Check sheet for the modelled part. Datum: model origin and axes. Units: mm. A direction names the side the tool comes from. Give positions to 0.01 mm unless a question says otherwise; leave off trailing zeros. Order: outer loops, then holes, each group sorted by start corner. A loop starts at its lowest first (then second) coordinate and runs counter-clockwise, first axis right, second up. Notation, with made-up numbers: M -3.75,19 L 15.25,19 A25 ccw 15.25,34 Z; hole C 75,8.5 d11. An arc over 180 degrees is marked long. One line per question, with ' | ' between items. Start each with the question number.
```python
from build123d import *

# Parameters (mm, degrees)
SKETCH_1_W          = 45
SKETCH_1_H          = 45
SKETCH_1_R          = 1.6
EXTRUDE_1_DEPTH     = 3
SKETCH_2_W          = 45
SKETCH_2_H          = 3
EXTRUDE_2_DEPTH     = 32
CUT_EXTRUDE_1_REACH = 61.626
SKETCH_3_R          = 4.1
FILLET_1_R          = 3
FILLET_2_R          = 8


with BuildPart() as part:
    # 草图1 → 凸台-拉伸1 (new body)
    with BuildSketch(Plane(origin=(0, 0, 0), x_dir=(1, 0, 0), z_dir=(0, 1, 0))):
        Rectangle(SKETCH_1_W, SKETCH_1_H)
        with Locations(Location((-17.5, -17.5, 0), (0, 0, 270))):
            Circle(SKETCH_1_R, mode=Mode.SUBTRACT)
        with Locations(Location((17.5, -17.5, 0), (0, 0, 270))):
            Circle(SKETCH_1_R, mode=Mode.SUBTRACT)
        with Locations(Location((17.5, 7.5, 0), (0, 0, 270))):
            Circle(SKETCH_1_R, mode=Mode.SUBTRACT)
        with Locations(Location((-17.5, 7.5, 0), (0, 0, 270))):
            Circle(SKETCH_1_R, mode=Mode.SUBTRACT)
    extrude(amount=EXTRUDE_1_DEPTH)

    # 草图2 → 凸台-拉伸2 (add)
    with BuildSketch(Plane.XZ):
        with Locations((0, -21)):
            Rectangle(SKETCH_2_W, SKETCH_2_H)
    extrude(amount=EXTRUDE_2_DEPTH)

    # 草图3 → 切除-拉伸1 (cut, up to next)
    with BuildSketch(Plane(origin=(0, 0, -22.5), x_dir=(-1, 0, 0), z_dir=(0, 0, -1)), mode=Mode.PRIVATE) as cut_extrude_1_sk1:
        with Locations((-14.5, -24)):
            Circle(SKETCH_3_R)
    cut_extrude_1_tool1 = extrude(cut_extrude_1_sk1.sketch, amount=-CUT_EXTRUDE_1_REACH, mode=Mode.PRIVATE) & part.part
    # 草图3 → 切除-拉伸1 (cut, up to next)
    with BuildSketch(Plane(origin=(0, 0, -22.5), x_dir=(-1, 0, 0), z_dir=(0, 0, -1)), mode=Mode.PRIVATE) as cut_extrude_1_sk2:
        with Locations((14.5, -24)):
            Circle(SKETCH_3_R)
    cut_extrude_1_tool2 = extrude(cut_extrude_1_sk2.sketch, amount=-CUT_EXTRUDE_1_REACH, mode=Mode.PRIVATE) & part.part
    add(cut_extrude_1_tool1.solids().sort_by_distance((14.5, -24, -22.5))[0], mode=Mode.SUBTRACT)
    add(cut_extrude_1_tool2.solids().sort_by_distance((-14.5, -24, -22.5))[0], mode=Mode.SUBTRACT)

    # 圆角1
    fillet_1_edges = [part.edges().sort_by_distance(p)[0] for p in [
        (22.5, 1.5, 22.5),
        (-22.5, 1.5, 22.5),
        (0, 3, -22.5),
    ]]
    fillet(fillet_1_edges, radius=FILLET_1_R)

    # 圆角2
    fillet_2_edges = [part.edges().sort_by_distance(p)[0] for p in [
        (22.5, -32, -21),
        (-22.5, -32, -21),
    ]]
    fillet(fillet_2_edges, radius=FILLET_2_R)


solid = part.part
```
Item 1: Scan lines: probe 1 along X at (y, z) = (1.95, -7.5); probe 2 along Z at (x, y) = (-13.5, -10); probe 3 along Y at (x, z) = (8, 0). Record each from-to range of solid material in increasing order. Write a range as [from, to].
Item 2: Section check B-B, the plane z = 17.5. Record the cut outline in (x, y), then the cut area to 3 significant figures.
Item 3: Go/stop test with flat-tipped pins: P1, Ø7.5, axis at x = -14.5, y = -24, coming from the -Z side; P2, Ø3.5, axis at x = 17.5, z = 17.5, coming from the -Y side; P3, Ø6, axis at x = -14.5, y = -11.5, coming from the +Z side. Record where each tip stops, or that it passes through.
Item 4: Section check D-D, the plane x = -8.5. Record the cut outline in (y, z), then the cut area to 3 significant figures.
Item 5: Draft check along Y on faces 1 (the face through (0, -32, -21)), 2 (the face through (0, -16, -22.5)), 3 (the face through (-11.246, -26.495, -21.021)). Enter one of: released by +Y, released by -Y, zero draft, split by the parting line, or undercut.
Item 6: Section check A-A, the plane x = 12. Record the cut outline in (y, z).
Item 7: Set-up check for faces 4 (the face through (0, 0, 1)), 5 (the face through (-22.5, 1, -9)): record each of +Z, -Z, +X, -X, +Y, -Y from which the full face is reachable in a straight line by a thin tool's end or side.
Item 8: Section check C-C, the plane y = -23. Record the cut outline in (x, z), then the cut area to 3 significant figures.
Reported:
1) probe 1: x = [-22.5, -19.1], [-15.9, 15.9], [19.1, 22.5] | probe 2: z = [-22.5, -19.5] | probe 3: y = [0, 3]
2) outline: M -22.5,0 L -19.1,0 L -19.1,3 L -22.5,3 Z; M -15.9,0 L 15.9,0 L 15.9,3 L -15.9,3 Z; M 19.1,0 L 22.5,0 L 22.5,3 L 19.1,3 Z | area: 116 mm^2
3) P1: passes through | P2: stops at y = 0 | P3: stops at z = -19.5
4) outline: M -32,-22.5 L 0,-22.5 A3 ccw 3,-19.5 L 3,22.5 L 0,22.5 L 0,-19.5 L -32,-19.5 Z | area: 229 mm^2
5) face 1: released by -Y | face 2: zero draft | face 3: undercut
6) outline: M -32,-22.5 L -27.25,-22.5 L -27.25,-19.5 L -32,-19.5 Z; M -20.75,-22.5 L 0,-22.5 A3 ccw 3,-19.5 L 3,22.5 L 0,22.5 L 0,-19.5 L -20.75,-19.5 Z
7) face 4: +Z, +X, -X, -Y | face 5: +Z, -Z, -X, +Y, -Y
8) outline: M -22.5,-22.5 L -18.48,-22.5 L -18.48,-19.5 L -22.5,-19.5 Z; M -10.52,-22.5 L 10.52,-22.5 L 10.52,-19.5 L -10.52,-19.5 Z; M 18.48,-22.5 L 22.5,-22.5 L 22.5,-19.5 L 18.48,-19.5 Z | area: 87.3 mm^2
